Job drawing, mm, ordinate dimensions from the low corner. One solid piece. A direction names the side the tool comes from. Round coordinates to 2 decimals unless told otherwise and drop trailing zeros. Write each loop counter-clockwise with the first axis right and the second up, starting at its lowest first coordinate (ties: lowest second). Pieces come first, ordered by that corner, then holes.
1) Drill centre lines: L1, parallel to X at y = 29, z = 25; L2, parallel to Z at x = 25, y = 28; L3, parallel to X at y = 7.5, z = 33. Where is each one in solid material? Low to high.
2) Which spindle directions (+Z, -Z, +X, -X, +Y, -Y) get a long thin tool onto all of the face, cutting with end or side? Do the marked faces 1, 2 and 3. Say none if no direction does.
3) Saw through at D-D on x = 93.5. Write the cut outline in (y, z).
4) Flat gauge pins, fed straight in: pin 1 (6 mm diameter, centred on x = 16, y = 19.5, fed in from +Z); pin 2 (6 mm diameter, centred on x = 91.5, z = 34, fed in from +Y); pin 3 (17 mm diameter, centred on x = 25.4, z = 25.4, fed in from -Y); pin 4 (10 mm diameter, centred on x = 126, y = 18, fed in from -Z). Where does each tip first touch, or does it go through?
5) Saw through at B-B on x = 47. Write the cut outline in (y, z).
6) Saw through at A-A on y = 25.4. Write the cut outline in (x, z) (3 decimals).
7) Saw through at C-C on y = 44. Write the cut outline in (x, z), and give its area (3 significant figures).
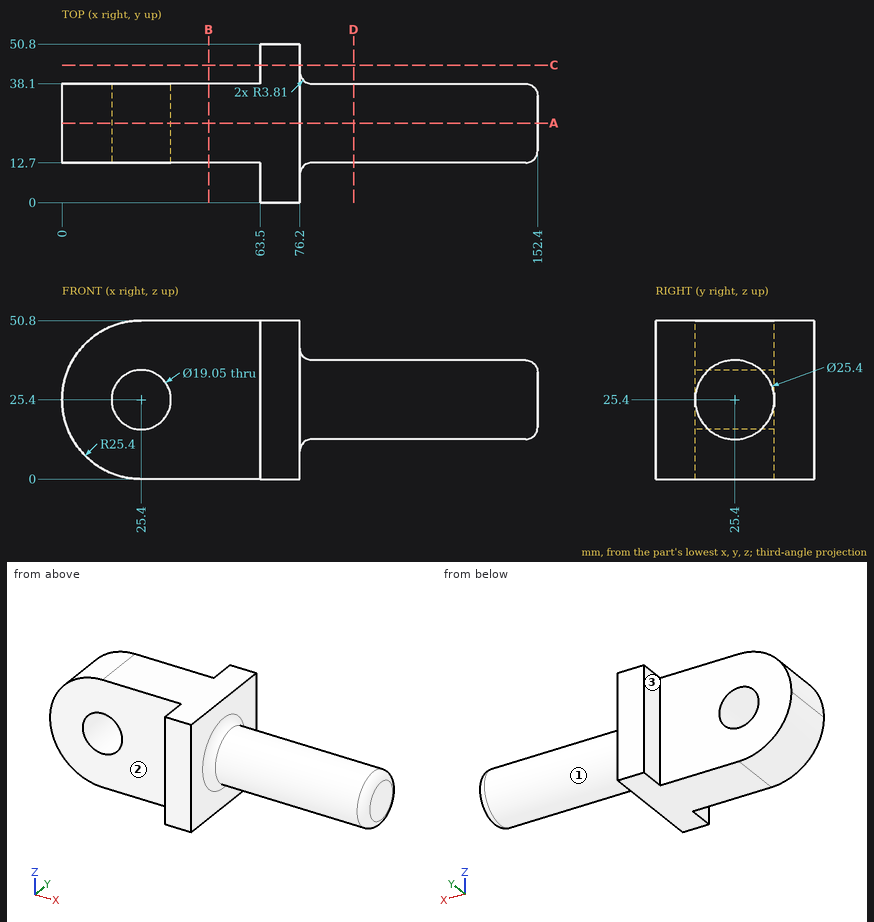
Completed:
1. L1: x = 0 to 15.88, 34.92 to 152.4
1. L2: z = 0 to 15.88, 34.92 to 50.8
1. L3: x = 63.5 to 76.2
2. face 1: +X
2. face 2: +Z, -Z, -X, -Y
2. face 3: +Z, -Z, -X, +Y
3. outline: circle Ø25.4 at (25.4, 25.4)
4. pin 1: stops at z = 49.98
4. pin 2: stops at y = 36.8
4. pin 3: passes through
4. pin 4: stops at z = 12.93
5. outline: (12.7, 0) - (38.1, 0) - (38.1, 50.8) - (12.7, 50.8) - close
6. outline: (0, 25.4) arc R25.4 ccw to (25.4, 0) - (76.2, 0) - (76.2, 8.89) arc R3.81 cw to (80.01, 12.7) - (148.59, 12.7) arc R3.81 ccw to (152.4, 16.51) - (152.4, 34.29) arc R3.81 ccw to (148.59, 38.1) - (80.01, 38.1) arc R3.81 cw to (76.2, 41.91) - (76.2, 50.8) - (25.4, 50.8) arc R25.4 ccw to start; hole circle Ø19.05 at (25.4, 25.4)
7. outline: (63.5, 0) - (76.2, 0) - (76.2, 50.8) - (63.5, 50.8) - close
7. area: 645 mm2
